from build123d import *

# Parameters (mm, degrees)
F0_W     = 152.4
F0_H     = 50.8
F1_DEPTH = 76.2
F3_DEPTH = 3.175


with BuildPart() as f1:
    # F0 (on Front) → F1 (new body)
    with BuildSketch(Plane.XZ):
        Rectangle(F0_W, F0_H)
    extrude(amount=F1_DEPTH)

    # F2 (on face) → F3 (cut)
    with BuildSketch(Plane.XZ.offset(76.2)):
        with BuildLine():
            ThreePointArc((-66.675, 0), (-50.8, -15.875), (-34.925, 0))
            ThreePointArc((-34.925, 0), (-50.8, 15.875), (-66.675, 0))
        make_face()
    extrude(amount=-F3_DEPTH, mode=Mode.SUBTRACT)


solid = f1.part
The listing builds one solid part. Answer for the finished solid, in the listing's coordinates (mm). Round coordinates to 2 decimals unless told otherwise and drop trailing zeros. Write each loop counter-clockwise with the first axis right and the second up, starting at its lowest first coordinate (ties: lowest second). Pieces come first, ordered by that corner, then holes. Notation, with made-up numbers: M 55,88.25 L 91,88.25 A8 ccw 91,94.25 Z; hole C 62,-32 d1. An arc over 180 degrees is marked long. Write each question's results on one line, items separated by ' | '. Start each with the question number.
Item 1: Given pin 1 Ø10 at (x, z) = (-11, -15) entering from +Y, flat-ended and moving along its own axis, determine where the tip first touches the part or whether it passes through.
Item 2: Find section A-A on x = -50.8. Write down the section's boundary in (y, z) (3 decimals).
Item 3: The mould has two halves that part along Z. Classify faces 1 (the cylindrical face through (-36.136, -74.635, -6.08)), 2 (the flat face through (-1, 0, 0)), 3 (the flat face through (-1, -38, 25.4)), 4 (the flat face through (-51, -73.025, 0)): +Z half, -Z half, draft (parallel to the pull), parting line (faces both ways), or undercut.
Item 4: A straight line is drawn through the part: probe 1 along Z at (x, y) = (-50, -74). Find the intervals that lie inside material, in ascending order.
Answer block:
1) pin 1: stops at y = 0
2) outline: M -76.2,-25.4 L 0,-25.4 L 0,25.4 L -76.2,25.4 L -76.2,15.875 L -73.025,15.875 L -73.025,-15.875 L -76.2,-15.875 Z
3) face 1: undercut | face 2: draft | face 3: +Z half | face 4: undercut
4) probe 1: z = -25.4 to -15.85, 15.85 to 25.4
